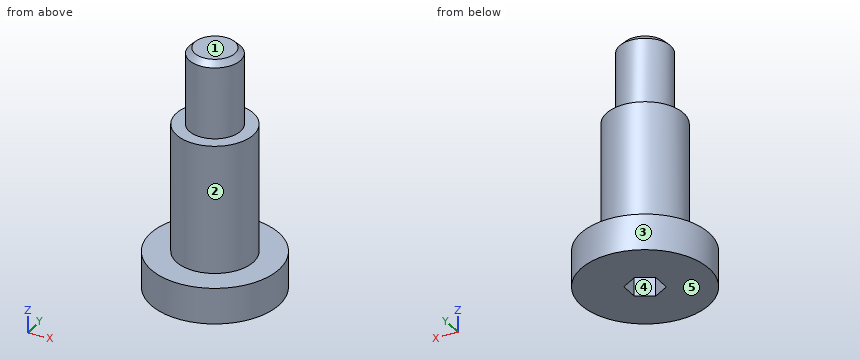
Autodesk Inventor part; units mm, degrees
ref_plane "YZ Plane" through (0, 0, 0) normal (1, 0, 0) x (0, 1, 0)
ref_plane "XZ Plane" through (0, 0, 0) normal (0, 1, 0) x (-1, 0, 0)
ref_plane "XY Plane" through (0, 0, 0) normal (0, 0, 1) x (1, 0, 0)
sketch "Sketch1" plane through (0, 0, 0) normal (0, 1, 0) x (-1, 0, 0)
  line L0 (0, 0) -> (0, 18.8)
  line L1 (0, 18.8) -> (-2, 18.8)
  line L2 (-2, 18.8) -> (-2, 12.8)
  line L3 (-2, 12.8) -> (-3, 12.8)
  line L4 (-3, 12.8) -> (-3, 2.8)
  line L5 (-3, 2.8) -> (-5, 2.8)
  line L6 (-5, 2.8) -> (-5, 0)
  line L7 (-5, 0) -> (0, 0)
  dimension "d0" = 10
  dimension "d1" = 6
  dimension "d2" = 4
  dimension "d3" = 6
  dimension "d4" = 10
  dimension "d5" = 2.8
revolve "Revolution1" add sketch "Sketch1" angle 360 about axis through (0, 0, 0) along (0, 0, 1)
thread "Thread1"
sketch "Sketch2" plane through (0, 0, 0) normal (0, 0, -1) x (-1, 0, 0)
  line L0 (0, 1.4434) -> (1.25, 0.7217)
  line L1 (1.25, 0.7217) -> (1.25, -0.7217)
  line L2 (1.25, -0.7217) -> (0, -1.4434)
  line L3 (0, -1.4434) -> (-1.25, -0.7217)
  line L4 (-1.25, -0.7217) -> (-1.25, 0.7217)
  line L5 (-1.25, 0.7217) -> (0, 1.4434)
  point P0 (0, 0)
  point P1 (0, 0)
  dimension "d9" = 2.5
extrude "Extrusion1" cut sketch "Sketch2" against normal blind 2
chamfer "Chamfer1" distance 0.43 angle 45 1 edges at (-2, 0, 18.8)
properties part number "DBSY4-10-6" material "Stainless Steel AISI 304"
Design review of the part built by this model. Coordinates are the model's own, in mm. Face numbers are marked on the shaded views. A direction names the side the tool comes from. Round coordinates to 2 decimals unless told otherwise and drop trailing zeros. Order: outer loops, then holes, each group sorted by start corner. A loop starts at its lowest first (then second) coordinate and runs counter-clockwise, first axis right, second up. Notation, with made-up numbers: (16.25, 78.25) - (63.25, 78.25) arc R22 ccw to (63.25, 95.25) - close; hole circle Ø5 at (-20.5, 13). An arc over 180 degrees is marked (long way). Return JSON: item names as keys, results as strings.
Q1. Consider section A-A on y = 0. Write out the cut boundary in (x, z), plus the area to 3 significant figures.
Computed values:
{"outline": "(-5, 0) - (-1.25, 0) - (-1.25, 2) - (1.25, 2) - (1.25, 0) - (5, 0) - (5, 2.8) - (3, 2.8) - (3, 12.8) - (2, 12.8) - (2, 18.37) - (1.57, 18.8) - (-1.57, 18.8) - (-2, 18.37) - (-2, 12.8) - (-3, 12.8) - (-3, 2.8) - (-5, 2.8) - close", "area": "107 mm2"}
Q2. Consider section C-C on x = 4. Write out the cut boundary in (y, z).
Computed values:
{"outline": "(-3, 0) - (3, 0) - (3, 2.8) - (-3, 2.8) - close"}
Q3. Consider section D-D on z = 16.25. Write out the cut boundary in (x, y), plus the area to 3 significant figures.
Computed values:
{"outline": "circle Ø4 at (0, 0)", "area": "12.6 mm2"}
Q4. Machinability: for the marked faces 1 and 2, which of the approach directions +Z, -Z, +X, -X, +Y, -Y give a long, thin tool a straight path to every point of the face, cutting with its end or side? Answer none if there is none.
Computed values:
{"face 1": "+Z, +X, -X, +Y, -Y", "face 2": "+Z"}
Q5. Consider section B-B on z = 8.5. Write out the cut boundary in (x, y), plus the area to 3 significant figures.
Computed values:
{"outline": "circle Ø6 at (0, 0)", "area": "28.3 mm2"}
Q6. Wall thickness on L1, parallel to Z at x = 1, y = 4; L2, parallel to Z at x = -2, y = -1; L3, parallel to X at y = 2.75, z = 6: over which ranges is each line inside the solid? List them lowest first. Write a range as [from, to].
Computed values:
{"L1": "z = [0, 2.8]", "L2": "z = [0, 12.8]", "L3": "x = [-1.2, 1.2]"}
Q7. For pin 1 Ø2 at (x, z) = (0.5, 4.5) entering from -Y; pin 2 Ø2 at (x, y) = (0, 0) entering from -Z; pin 3 Ø5 at (x, z) = (2.5, 4.5) entering from -Y, all flat-tipped, find the tip position at first contact; note any pin that passes through.
Computed values:
{"pin 1": "stops at y = -3", "pin 2": "stops at z = 2", "pin 3": "stops at y = -4.96"}
Q8. The part is to be moulded in two halves that separate along X. For the marked faces 3, 4 and 5, say which applies: pulls with the +X half, pulls with the -X half, needs draft (parallel to the pull), parting line crosses it, or undercut.
Computed values:
{"face 3": "parting line crosses it", "face 4": "undercut", "face 5": "needs draft"}
